```python
from build123d import *

# Parameters (mm, degrees)
BOSS_EXTRU_1_DEPTH      = 15
ESQUISSE2_W             = 42
ESQUISSE2_H             = 22
ENL_V_MAT_EXTRU_1_DEPTH = 48.360320945
ESQUISSE4_R             = 2.15
ENL_V_MAT_EXTRU_2_DEPTH = 3
ESQUISSE5_W             = 4
ESQUISSE5_H             = 6.35
ENL_V_MAT_EXTRU_3_DEPTH = 6
ESQUISSE6_W             = 4
ESQUISSE6_H             = 6.35
ENL_V_MAT_EXTRU_4_DEPTH = 8
BOSS_EXTRU_2_DEPTH      = 5
BOSS_EXTRU_2_DEPTH_BACK = 5
CHANFREIN1_SIZE         = 3
BOSS_EXTRU_4_DEPTH      = 5
BOSS_EXTRU_6_START      = 20
ESQUISSE13_W            = 12.5
ESQUISSE13_H            = 10
BOSS_EXTRU_6_DEPTH      = 20
ESQUISSE14_W            = 42
ESQUISSE14_H            = 10
BOSS_EXTRU_7_DEPTH      = 5
BOSS_EXTRU_8_START      = -5
BOSS_EXTRU_8_DEPTH      = 5
ESQUISSE17_R            = 4.5
ENL_V_MAT_EXTRU_5_DEPTH = 127.873828497


with BuildPart() as part:
    # Esquisse1 → Boss.-Extru.1 (new body)
    with BuildSketch(Plane.XY):
        with BuildLine():
            Line((30, -13), (-30, -13))
            Line((-30, -13), (-30, 13))
            Line((-30, 13), (30, 13))
            ThreePointArc((30, 13), (43, 0), (30, -13))
        make_face()
    extrude(amount=BOSS_EXTRU_1_DEPTH)

    # Esquisse2 → Enlèv. mat.-Extru.1 (cut, through all)
    with BuildSketch(Plane.XY.offset(15)):
        with Locations((3, 0)):
            Rectangle(ESQUISSE2_W, ESQUISSE2_H)
    extrude(amount=-ENL_V_MAT_EXTRU_1_DEPTH, mode=Mode.SUBTRACT)

    # Esquisse4 → Enlèv. mat.-Extru.2 (cut)
    with BuildSketch(Plane.XY.offset(15)):
        with Locations((-20.81, 4.935)):
            Circle(ESQUISSE4_R)
        with Locations((-20.81, -4.935)):
            Circle(ESQUISSE4_R)
        with Locations((28.49, 4.935)):
            Circle(ESQUISSE4_R)
        with Locations((28.49, -4.935)):
            Circle(ESQUISSE4_R)
    extrude(amount=-ENL_V_MAT_EXTRU_2_DEPTH, mode=Mode.SUBTRACT)

    # Esquisse5 → Enlèv. mat.-Extru.3 (cut)
    with BuildSketch(Plane(origin=(-18, 0, 0), x_dir=(0, 0, -1), z_dir=(1, 0, 0))):
        with Locations((-10, -4.825)):
            Rectangle(ESQUISSE5_W, ESQUISSE5_H)
        with Locations((-10, 4.825)):
            Rectangle(ESQUISSE5_W, ESQUISSE5_H)
    extrude(amount=-ENL_V_MAT_EXTRU_3_DEPTH, mode=Mode.SUBTRACT)

    # Esquisse6 → Enlèv. mat.-Extru.4 (cut)
    with BuildSketch(Plane.ZY.offset(-24)):
        with Locations((10, 4.825)):
            Rectangle(ESQUISSE6_W, ESQUISSE6_H)
        with Locations((10, -4.825)):
            Rectangle(ESQUISSE6_W, ESQUISSE6_H)
    extrude(amount=-ENL_V_MAT_EXTRU_4_DEPTH, mode=Mode.SUBTRACT)

    # Esquisse9 → Boss.-Extru.2 (add, two sides: drawn at the far end of the back side and taken through both)
    with BuildSketch(Plane.XY.offset(7.5).offset(-BOSS_EXTRU_2_DEPTH_BACK)):
        Polygon((-30, 33), (-95, 33), (-95, 28), (-35, 28), (-35, 0), (-35, -23), (-95, -23), (-95, -28), (-30, -28), (-30, 0), align=None)
    extrude(amount=BOSS_EXTRU_2_DEPTH + BOSS_EXTRU_2_DEPTH_BACK)

    # Chanfrein1
    # the kernel refuses this chamfer: 3 mm, written as the material it adds along each edge
    with BuildSketch(Plane(origin=(-30, 13, 12.5), x_dir=(0.02749587661058678, 0, 0.9996219169112968), z_dir=(0, -1, 0))) as chanfrein1_piece_1_section:
        Polygon((CHANFREIN1_SIZE * 0.999621916911, CHANFREIN1_SIZE * 0.0274958766106), (-CHANFREIN1_SIZE * 0.0274958766106, CHANFREIN1_SIZE * 0.999621916911), (0, 0), align=None)
    chanfrein1_piece_1 = extrude(amount=26, mode=Mode.PRIVATE)
    chanfrein1_piece_1 = split(chanfrein1_piece_1, bisect_by=Plane(origin=(-31.023809524, 0, 15), z_dir=(0, 0, -1)), keep=Keep.TOP, mode=Mode.PRIVATE)
    add(chanfrein1_piece_1)
    with BuildSketch(Plane(origin=(-30, -13, 2.5), x_dir=(0.027495876610585626, 0, -0.9996219169112968), z_dir=(0, 1, 0))) as chanfrein1_piece_2_section:
        Polygon((CHANFREIN1_SIZE * 0.999621916911, CHANFREIN1_SIZE * 0.0274958766106), (-CHANFREIN1_SIZE * 0.0274958766106, CHANFREIN1_SIZE * 0.999621916911), (0, 0), align=None)
    chanfrein1_piece_2 = extrude(amount=26, mode=Mode.PRIVATE)
    chanfrein1_piece_2 = split(chanfrein1_piece_2, bisect_by=Plane(origin=(-31.023809524, 0, 0), z_dir=(0, 0, 1)), keep=Keep.TOP, mode=Mode.PRIVATE)
    add(chanfrein1_piece_2)

    # Esquisse11 → Boss.-Extru.4 (add)
    with BuildSketch(Plane.XZ.offset(28)):
        with BuildLine():
            Line((-95, 2.5), (-95, 12.5))
            Line((-95, 12.5), (-104.43476759, 12.5))
            ThreePointArc((-104.43476759, 12.5), (-109.43476759, 7.5), (-104.43476759, 2.5))
            Line((-104.43476759, 2.5), (-95, 2.5))
        make_face()
    extrude(amount=-BOSS_EXTRU_4_DEPTH)

    # Esquisse13 → Boss.-Extru.6 (add)
    with BuildSketch(Plane(origin=(0, 0, 0), x_dir=(-1, 0, 0), z_dir=(0, 0, -1)).offset(BOSS_EXTRU_6_START)):
        with BuildLine():
            Line((-24, -5), (-24, 5))
            Line((-24, 5), (-42, 5))
            ThreePointArc((-42, 5), (-43, 0), (-42, -5))
            Line((-42, -5), (-24, -5))
        make_face()
        with Locations((24.25, 0)):
            Rectangle(ESQUISSE13_W, ESQUISSE13_H)
    extrude(amount=-BOSS_EXTRU_6_DEPTH)

    # Esquisse14 → Boss.-Extru.7 (add)
    with BuildSketch(Plane(origin=(0, 0, -20), x_dir=(-1, 0, 0), z_dir=(0, 0, -1))):
        with Locations((-3, 0)):
            Rectangle(ESQUISSE14_W, ESQUISSE14_H)
    extrude(amount=-BOSS_EXTRU_7_DEPTH)

    # Esquisse16 → Boss.-Extru.8 (add)
    with BuildSketch(Plane(origin=(0, 33, 0), x_dir=(1, 0, 0), z_dir=(0, 1, 0)).offset(BOSS_EXTRU_8_START)):
        with BuildLine():
            Line((-89.416041875, -12.5), (-104.43476759, -12.5))
            ThreePointArc((-104.43476759, -12.5), (-109.43476759, -7.5), (-104.43476759, -2.5))
            Line((-104.43476759, -2.5), (-89.416041875, -2.5))
            Line((-89.416041875, -2.5), (-89.416041875, -12.5))
        make_face()
    extrude(amount=BOSS_EXTRU_8_DEPTH)

    # Esquisse17 → Enlèv. mat.-Extru.5 (cut, through all)
    with BuildSketch(Plane.XZ.offset(28)):
        with Locations((-95, 7.5)):
            Circle(ESQUISSE17_R)
    extrude(amount=-ENL_V_MAT_EXTRU_5_DEPTH, mode=Mode.SUBTRACT)


solid = part.part
```
Model file for the job. Use its own axes, mm. A direction names the side the tool comes from. Give positions to 0.01 mm unless a question says otherwise; leave off trailing zeros. Loops run counter-clockwise (first coordinate to the right, second up) from the corner with the lowest first, then second, coordinate; pieces in that order, holes last. Notation, with made-up numbers: (61.5, 66.5) -> (78.5, 66.5) arc R14 ccw to (78.5, 91.5) -> close; hole circle Ø11 at (4, 30). An arc over 180 degrees is marked (long way). Use CSV: the item, a comma, the result in double quotes. Start each with the question number.
1) Slice it at A-A on x = 20.5. Give the cut face in (y, z), plus the area to 3 significant figures.
2) Slice it at B-B on x = -83. Give the cut face in (y, z), plus the area to 3 significant figures.
3) Slice it at C-C on z = -7. Give the cut face in (x, y).
4) Slice it at D-D on y = 0. Give the cut face in (x, z).
5) Wall check: line 1 (Y direction, x = -20.81, z = 13.75) (3 decimals); line 2 (Z direction, x = -95, y = -25.1); line 3 (Y direction, x = -56, z = 8). Give the ranges that are in metal, low to high.
6) Tool access for faces 4 (the cylindrical face through (26.342, -4.84, 13.521)), 5 (the flat face through (-21, -5, 8)), 6 (the flat face through (-73, 28, 7)): list every direction of +Z, -Z, +X, -X, +Y, -Y with a clear straight run to the whole face (end or side of a thin tool).
7) Mould opens along Z. For faces 1 (the cylindrical face through (-99.496, -25.535, 7.698)), 2 (the flat face through (-18, 0, 4)), 3 (the flat face through (-62, -25, 2.5)) say: released by +Z, released by -Z, zero draft, split by the parting line, or undercut.
8) Flat gauge pins, fed straight in: pin 1 Ø11.5 at (x, z) = (-95, 7.5) entering from -Y; pin 2 Ø12 at (x, z) = (10, 7) entering from -Y; pin 3 Ø3 at (y, z) = (25.5, 7) entering from +X; pin 4 Ø7.5 at (x, z) = (7, 4) entering from +Y. Where does each tip first touch, or does it go through?
Computed values:
1,outline,"(-13, 0) -> (-11, 0) -> (-11, 15) -> (-13, 15) -> close; (-5, -20) -> (5, -20) -> (5, -15) -> (-5, -15) -> close; (11, 0) -> (13, 0) -> (13, 15) -> (11, 15) -> close"
1,area,"110 mm^2"
2,outline,"(-28, 2.5) -> (-23, 2.5) -> (-23, 12.5) -> (-28, 12.5) -> close; (28, 2.5) -> (33, 2.5) -> (33, 12.5) -> (28, 12.5) -> close"
2,area,"100 mm^2"
3,outline,"(-30.5, -5) -> (-18, -5) -> (-18, 5) -> (-30.5, 5) -> close; (24, -5) -> (42, -5) arc R13 ccw to (42, 5) -> (24, 5) -> close"
4,outline,"(-35, 2.5) -> (-33, 2.5) -> (-30.5, 0) -> (-30.5, -20) -> (43, -20) -> (43, 15) -> (24, 15) -> (24, -15) -> (-18, -15) -> (-18, 15) -> (-30.5, 15) -> (-33, 12.5) -> (-35, 12.5) -> close"
5,line 1,"y = -13 to -7.085, -2.785 to 2.785, 7.085 to 13"
5,line 2,"z = 2.5 to 3, 12 to 12.5"
5,line 3,"y = -28 to -23, 28 to 33"
6,face 4,"+Z"
6,face 5,"none"
6,face 6,"+Z, -Z, -X"
7,face 1,"undercut"
7,face 2,"zero draft"
7,face 3,"released by -Z"
8,pin 1,"stops at y = -28"
8,pin 2,"stops at y = -13"
8,pin 3,"stops at x = -30"
8,pin 4,"stops at y = 13"
